CAD build for the part. Positions are in the model's coordinates, mm. Face numbers are marked on the shaded views. A direction names the side the tool comes from. Give positions to 0.01 mm unless a question says otherwise; leave off trailing zeros. Loops run counter-clockwise (first coordinate to the right, second up) from the corner with the lowest first, then second, coordinate; pieces in that order, holes last.
Item 1: Saw through at B-B on x = 0. Give the cut face in (y, z) (3 decimals).
Item 2: Probe probe 1 along Y at (x, z) = (0, 3); probe 2 along X at (y, z) = (13.25, 6); probe 3 along X at (y, z) = (-3.25, 13.5). List the from-to ranges inside material, lowest first.
Item 3: Saw through at C-C on z = 3. Give the cut face in (x, y).
Item 4: Which spindle directions (+Z, -Z, +X, -X, +Y, -Y) get a long thin tool onto all of the face, cutting with end or side? Do the marked faces 4, 5, 6, 7 and 8. Say none if no direction does.
Item 5: Mould opens along Y. For the marked faces 1, 2 and 3 say: released by +Y, released by -Y, zero draft, split by the parting line, or undercut.
Item 6: Saw through at D-D on y = -10. Give the cut face in (x, z), plus the area to 3 significant figures.
Item 7: Saw through at A-A on y = 6.25. Give the cut face in (x, z), plus the area to 3 significant figures.
Item 8: Drop flat-ended pins along their axis: P1, Ø0.9, axis at x = 17, z = 7.5, coming from the +Y side (3 decimals); P2, Ø3.5, axis at x = 0, z = 7.493, coming from the -Y side; P3, Ø1, axis at x = -9.5, z = 10.5, coming from the -Y side; P4, Ø4, axis at x = 8, y = 3, coming from the -Z side. Give the stop position or say it passes through.
from build123d import *

# Parameters (mm, degrees)
SKETCH1_W               = 35.052
SKETCH1_H               = 29.972
EXTRUDE1_DEPTH          = 14.986
CUT_EXTRUDE1_DEPTH      = 15.986
SKETCH3_W               = 2.27457
SKETCH3_H               = 9.990666667
CUT_EXTRUDE2_DEPTH      = 18.526
CUT_EXTRUDE2_DEPTH_BACK = 18.526
SKETCH4_W               = 33.4645
SKETCH4_H               = 13.3985
CUT_EXTRUDE3_DEPTH      = 0.254
SKETCH5_W               = 1.731382872
SKETCH5_H               = 7.88543
CUT_EXTRUDE4_DEPTH      = 1.651
EXTRUDE2_DEPTH          = 0.635


with BuildPart() as part:
    # Sketch1 → Extrude1 (new body)
    with BuildSketch(Plane.XY):
        Rectangle(SKETCH1_W, SKETCH1_H)
    extrude(amount=EXTRUDE1_DEPTH)

    # Sketch2 → Cut-Extrude1 (cut, through all)
    with BuildSketch(Plane.XY.offset(14.986)):
        with BuildLine():
            Line((-11.684, 4.995333333), (-11.45032, 4.995333333))
            ThreePointArc((-11.45032, 4.995333333), (-11.673292179, 7.650930846), (-11.1204375, 10.257895833))
            Line((-11.1204375, 10.257895833), (-11.1204375, 13.758333333))
            Line((-11.1204375, 13.758333333), (-14.620875, 14.986))
            Line((-14.620875, 14.986), (14.620875, 14.986))
            Line((14.620875, 14.986), (11.1204375, 13.758333333))
            Line((11.1204375, 13.758333333), (11.1204375, 10.257895833))
            ThreePointArc((11.1204375, 10.257895833), (11.673292179, 7.650930846), (11.45032, 4.995333333))
            Line((11.45032, 4.995333333), (11.684, 4.995333333))
            ThreePointArc((11.684, 4.995333333), (0, -6.688666667), (-11.684, 4.995333333))
        make_face()
    extrude(amount=-CUT_EXTRUDE1_DEPTH, mode=Mode.SUBTRACT)

    # Sketch3 → Cut-Extrude2 (cut, two sides)
    with BuildSketch(Plane(origin=(0, 0, 0), x_dir=(0, 0, -1), z_dir=(1, 0, 0))) as cut_extrude2_sk:
        with Locations((-13.848715, 9.990666667)):
            Rectangle(SKETCH3_W, SKETCH3_H)
        with Locations((-1.137285, 9.990666667)):
            Rectangle(SKETCH3_W, SKETCH3_H)
    extrude(amount=CUT_EXTRUDE2_DEPTH, mode=Mode.SUBTRACT)
    extrude(cut_extrude2_sk.sketch, amount=-CUT_EXTRUDE2_DEPTH_BACK, mode=Mode.SUBTRACT)

    # Sketch4 → Cut-Extrude3 (cut)
    with BuildSketch(Plane.XZ.offset(14.986)):
        with Locations((0, 7.493)):
            Rectangle(SKETCH4_W, SKETCH4_H)
    extrude(amount=-CUT_EXTRUDE3_DEPTH, mode=Mode.SUBTRACT)

    # Sketch5 → Cut-Extrude4 (cut)
    with BuildSketch(Plane(origin=(0, 14.986, 0), x_dir=(1, 0, 0), z_dir=(0, 1, 0))):
        with Locations((-16.660308564, -7.493)):
            Rectangle(SKETCH5_W, SKETCH5_H)
        with Locations((16.660308564, -7.493)):
            Rectangle(SKETCH5_W, SKETCH5_H)
    extrude(amount=-CUT_EXTRUDE4_DEPTH, mode=Mode.SUBTRACT)

    # Sketch6 → Cut-Revolve1 (revolve, cut)
    with BuildSketch(Plane(origin=(0, 0, 7.493), x_dir=(-1, 0, 0), z_dir=(0, 0, -1)), mode=Mode.PRIVATE) as cut_revolve1_sk:
        Polygon((3.048, -14.732), (0, -14.732), (0, -8.636), (5.969, -8.636), (5.969, -11.684), (3.048, -11.684), align=None)
    revolve(cut_revolve1_sk.sketch.rotate(Axis((0, 0, 7.493), (0, -1, 0)), 270), axis=Axis((0, 0, 7.493), (0, -1, 0)), mode=Mode.SUBTRACT)  # turned: the seam where the file's is

    # Sketch7 → Extrude2 (add, symmetric)
    with BuildSketch(Plane(origin=(0, 0, 7.493), x_dir=(-1, 0, 0), z_dir=(0, 0, -1))):
        with BuildLine():
            Line((4.641424464, -4.216434167), (8.676143507, -0.583556822))
            Line((8.676143507, -0.583556822), (9.621541413, -1.633527567))
            ThreePointArc((9.621541413, -1.633527567), (7.818122005, -3.687570808), (5.586822369, -5.266404912))
            Line((5.586822369, -5.266404912), (4.641424464, -4.216434167))
        make_face()
        with BuildLine():
            Line((-4.641424464, -4.216434167), (-5.586822369, -5.266404912))
            ThreePointArc((-5.586822369, -5.266404912), (-7.818122005, -3.687570808), (-9.621541413, -1.633527567))
            Line((-9.621541413, -1.633527567), (-8.676143507, -0.583556822))
            Line((-8.676143507, -0.583556822), (-4.641424464, -4.216434167))
        make_face()
    extrude(amount=EXTRUDE2_DEPTH, both=True)


solid = part.part
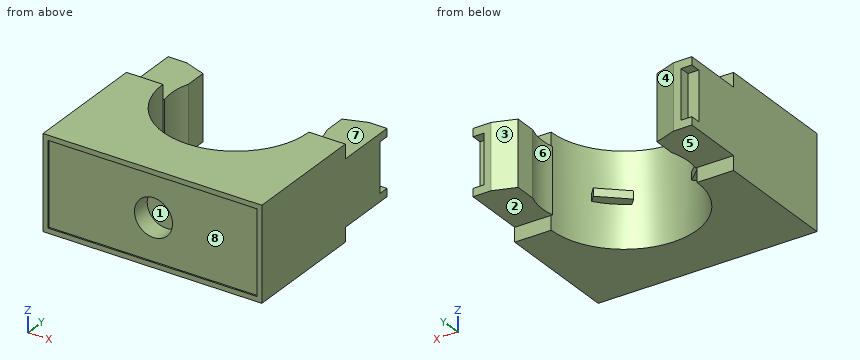
Results below:
1. outline: (-14.986, 0) - (-6.689, 0) - (-6.689, 14.986) - (-14.986, 14.986) - (-14.986, 14.192) - (-14.732, 14.192) - (-14.732, 10.541) - (-11.684, 10.541) - (-11.684, 13.462) - (-8.636, 13.462) - (-8.636, 1.524) - (-11.684, 1.524) - (-11.684, 4.445) - (-14.732, 4.445) - (-14.732, 0.794) - (-14.986, 0.794) - close
2. probe 1: y = -14.73 to -11.68, -8.64 to -6.69
2. probe 2: x = -17.53 to -11.12, 11.12 to 17.53
2. probe 3: x = -17.53 to -8.28, 8.28 to 17.53
3. outline: (-17.53, -14.99) - (-16.73, -14.99) - (-16.73, -14.73) - (16.73, -14.73) - (16.73, -14.99) - (17.53, -14.99) - (17.53, 14.99) - (14.62, 14.99) - (11.12, 13.76) - (11.12, 10.26) arc R9.14 cw to (11.45, 5) - (11.68, 5) arc R11.68 cw to (-11.68, 5) - (-11.45, 5) arc R9.14 cw to (-11.12, 10.26) - (-11.12, 13.76) - (-14.62, 14.99) - (-17.53, 14.99) - close; hole (-3.93, -11.68) - (3.93, -11.68) - (3.93, -8.64) - (-3.93, -8.64) - close
4. face 4: +Z, -Z, +Y
4. face 5: -Z, +X, -X, +Y
4. face 6: +Z, -Z
4. face 7: +Z, +X, -X, +Y
4. face 8: -Y
5. face 1: undercut
5. face 2: zero draft
5. face 3: released by +Y
6. outline: (-17.53, 0) - (17.53, 0) - (17.53, 14.99) - (-17.53, 14.99) - close; hole circle Ø11.94 at (0, 7.49)
6. area: 413 mm2
7. outline: (-17.53, 2.27) - (-11.65, 2.27) - (-11.65, 12.71) - (-17.53, 12.71) - close; (11.65, 2.27) - (17.53, 2.27) - (17.53, 12.71) - (11.65, 12.71) - close
7. area: 123 mm2
8. P1: stops at y = 13.335
8. P2: stops at y = -8.64
8. P3: stops at y = -14.73
8. P4: passes through
